```python
from build123d import *

# Parameters (mm, degrees)
F1_DEPTH = 177.8
F4_DEPTH = 25.4


with BuildPart() as f1:
    # F0 (on Front) → F1 (new body)
    with BuildSketch(Plane.XZ):
        Polygon((0, 82.55), (0, 0), (25.4, 0), (25.4, 5.08), (5.08, 5.08), (5.08, 82.55), align=None)
    extrude(amount=F1_DEPTH)

    # F3 (on face) → F4 (cut)
    with BuildSketch(Plane(origin=(0, 0, 0), x_dir=(0, -1, 0), z_dir=(-1, 0, 0))):
        with BuildLine():
            ThreePointArc((0, 69.85), (7.505978, 81.439311), (21.151517, 79.32955))
            Line((21.151517, 79.32955), (76.222725, 30.230675))
            ThreePointArc((76.222725, 30.230675), (88.9, 25.4), (101.577275, 30.230675))
            Line((101.577275, 30.230675), (156.648483, 79.32955))
            ThreePointArc((156.648483, 79.32955), (170.294022, 81.439311), (177.8, 69.85))
            Line((177.8, 69.85), (203.2, 69.85))
            Line((203.2, 69.85), (203.2, 95.25))
            Line((203.2, 95.25), (-25.4, 95.25))
            Line((-25.4, 95.25), (-25.4, 69.85))
            Line((-25.4, 69.85), (0, 69.85))
        make_face()
    extrude(amount=-F4_DEPTH, mode=Mode.SUBTRACT)


solid = f1.part
```
For this review, take the finished solid that the model builds, in its own axes (mm). A direction names the side the tool comes from. Coordinates: 2 decimals unless noted, no trailing zeros. Write each loop counter-clockwise with the first axis right and the second up, starting at its lowest first coordinate (ties: lowest second). Pieces come first, ordered by that corner, then holes. Notation, with made-up numbers: (83.25, 59.5) - (109.25, 59.5) arc R33 cw to (109.25, 94.5) - close; hole circle Ø2 at (3, 81). An arc over 180 degrees is marked (long way). Answer in a Markdown table with one row per item. Add a question column.
Q1. We need section C-C, the plane z = 20.5. State the section outline as (x, y) points.
Q2. Tool access review of faces 5 (the flat face through (15, -88, 5.08)), 6 (the flat face through (13, -88, 0)), 7 (the flat face through (2.504, -48.302, 55.124)): name each direction out of +Z, -Z, +X, -X, +Y, -Y from which nothing blocks a thin tool from reaching the whole face with its end or side.
Q3. For probe 1 along Z at (x, y) = (15.25, -16.5); probe 2 along Z at (x, y) = (3.5, -145.5), list the stretches that pass through material, from the lowest coordinate up.
Q4. We need section B-B, the plane y = -144. State the section outline as (x, z) points.
Q5. We need section A-A, the plane z = 36.5. State the section outline as (x, y) points, and give its area (3 significant figures).
Q6. We need section D-D, the plane x = 10.5. State the section outline as (y, z) points.
Q7. For P1, Ø1.5, axis at y = -101, z = 16, coming from the +X side; P2, Ø1, axis at x = 9, y = -18.5, coming from the +Z side; P3, Ø4, axis at x = 8, z = 8.5, coming from the -Y side, all flat-tipped, find the tip position at first contact; note any pin that passes through.
Q8. Draft analysis for pull direction Y (two halves, no side actions). For faces 1 (the flat face through (2.5, -128.73, 54.44)), 2 (the flat face through (4, -177.8, 27)), 3 (the flat face through (5.08, -88, 17)), 4 (the flat face through (4, 0, 27)), state which applies: +Y half, -Y half, draft (parallel to the pull), parting line (faces both ways), or undercut.
Answer list:
| question | item | result |
|---|---|---|
| 1 | outline | (0, -177.8) - (5.08, -177.8) - (5.08, 0) - (0, 0) - close |
| 2 | face 5 | +Z, +X, +Y, -Y |
| 2 | face 6 | -Z, +X, -X, +Y, -Y |
| 2 | face 7 | +Z, +X, -X |
| 3 | probe 1 | z = 0 to 5.08 |
| 3 | probe 2 | z = 0 to 69.39 |
| 4 | outline | (0, 0) - (25.4, 0) - (25.4, 5.08) - (5.08, 5.08) - (5.08, 68.05) - (0, 68.05) - close |
| 5 | outline | (0, -177.8) - (5.08, -177.8) - (5.08, -108.61) - (0, -108.61) - close; (0, -69.19) - (5.08, -69.19) - (5.08, 0) - (0, 0) - close |
| 5 | area | 703 mm2 |
| 6 | outline | (-177.8, 0) - (0, 0) - (0, 5.08) - (-177.8, 5.08) - close |
| 7 | P1 | stops at x = 5.08 |
| 7 | P2 | stops at z = 5.08 |
| 7 | P3 | passes through |
| 8 | face 1 | undercut |
| 8 | face 2 | -Y half |
| 8 | face 3 | draft |
| 8 | face 4 | +Y half |
